Check sheet for the drawn part. Datum: minimum x, y, z corner. Units: mm. Coordinates: 2 decimals unless noted, no trailing zeros. Order: outer loops, then holes, each group sorted by start corner. A loop starts at its lowest first (then second) coordinate and runs counter-clockwise, first axis right, second up.
1. Cross-section at B-B (y = 0.5). Enter the section's corners in (x, z).
2. Cross-section at A-A (z = 16.5). Enter the section's corners in (x, y).
3. Cross-section at C-C (x = 18). Enter the section's corners in (y, z), then the cut area to 3 significant figures.
4. Draft check along X on the marked faces 1, 2, 3 and 4. Enter one of: released by +X, released by -X, zero draft, split by the parting line, or undercut.
5. Cross-section at D-D (x = 14.25). Enter the section's corners in (y, z).
6. Thickness scan on line 1 (X direction, y = 2.05, z = 18.25); line 2 (Z direction, x = 14.25, y = 2.6); line 3 (Z direction, x = 7, y = 0.8). Record the ranges inside material, lowest first.
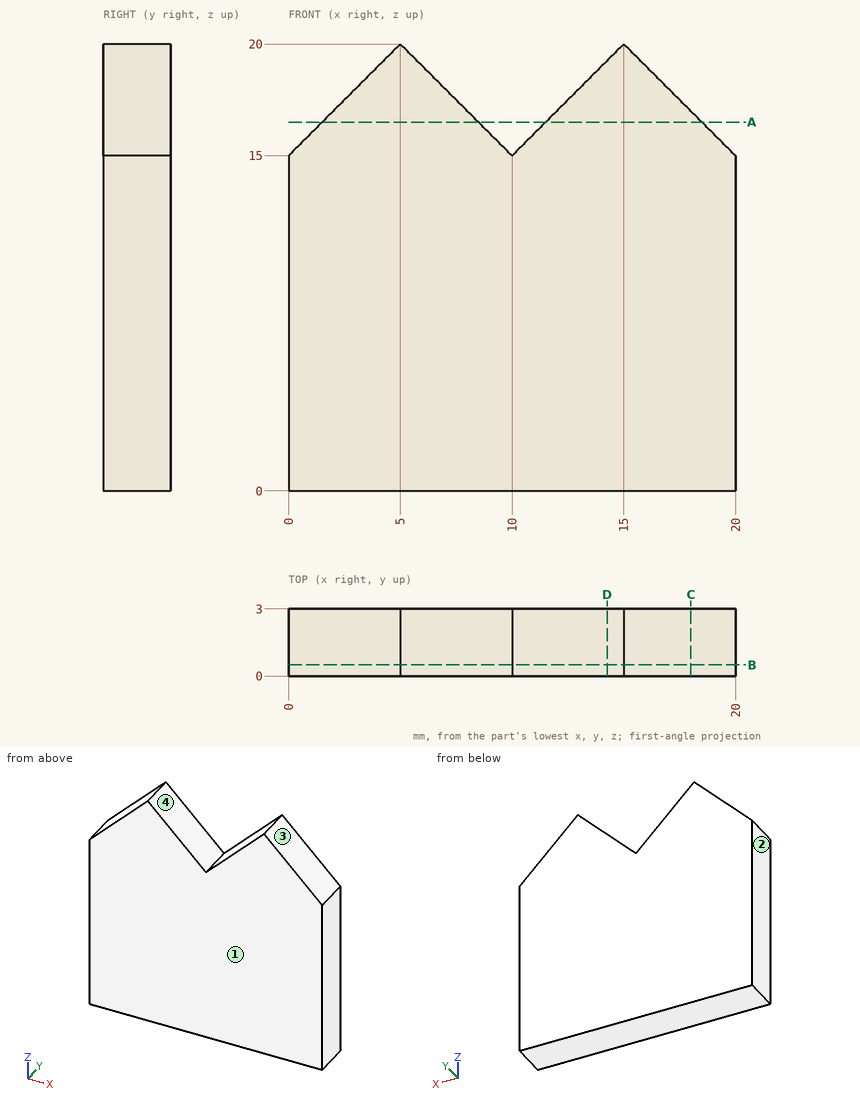
Data:
1. outline: (0, 0) - (20, 0) - (20, 15) - (15, 20) - (10, 15) - (5, 20) - (0, 15) - close
2. outline: (1.5, 0) - (8.5, 0) - (8.5, 3) - (1.5, 3) - close; (11.5, 0) - (18.5, 0) - (18.5, 3) - (11.5, 3) - close
3. outline: (0, 0) - (3, 0) - (3, 17) - (0, 17) - close
3. area: 51.0 mm2
4. face 1: zero draft
4. face 2: released by -X
4. face 3: released by +X
4. face 4: undercut
5. outline: (0, 0) - (3, 0) - (3, 19.25) - (0, 19.25) - close
6. line 1: x = 3.25 to 6.75, 13.25 to 16.75
6. line 2: z = 0 to 19.25
6. line 3: z = 0 to 18
